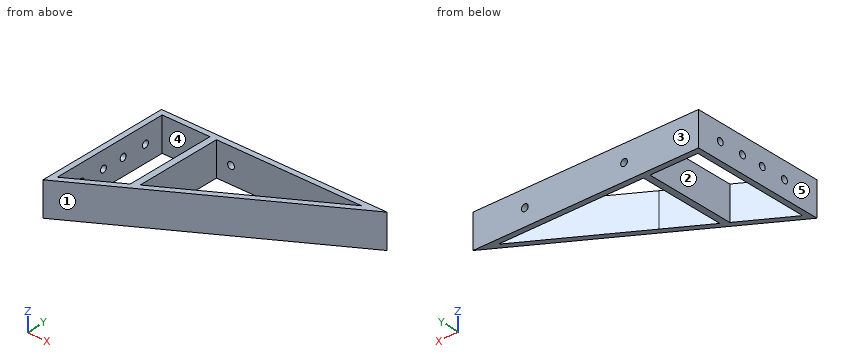
from build123d import *

# Parameters (mm, degrees)
F0_W     = 200
F0_H     = 120
F1_DEPTH = 30
F3_DEPTH = 30
F5_DEPTH = 30
F7_DEPTH = 6
F9_DEPTH = 6


with BuildPart() as f1:
    # F0 (on Top) → F1 (new body)
    with BuildSketch(Plane.XY):
        with Locations((-100, 60)):
            Rectangle(F0_W, F0_H)
    extrude(amount=F1_DEPTH)

    # F2 (on face) → F3 (cut)
    with BuildSketch(Plane.XY.offset(30)):
        Polygon((0, 120), (-200, 0), (0, 0), align=None)
    extrude(amount=-F3_DEPTH, mode=Mode.SUBTRACT)

    # F4 (on face) → F5 (cut)
    with BuildSketch(Plane.XY.offset(30)):
        Polygon((-195, 60.924411), (-195, 8.830952), (-152.64377, 34.24469), (-152.64377, 115), (-195, 115), align=None)
        Polygon((-146.821752, 115), (-146.821752, 37.737901), (-111.472848, 58.947243), (-18.051586, 115), (-115.799665, 115), align=None)
    extrude(amount=-F5_DEPTH, mode=Mode.SUBTRACT)

    # F6 (on face) → F7 (cut)
    with BuildSketch(Plane(origin=(0, 120, 0), x_dir=(-1, 0, 0), z_dir=(0, 1, 0))):
        with BuildLine():
            ThreePointArc((137, 15), (134, 18), (131, 15))
            ThreePointArc((131, 15), (134, 12), (137, 15))
        make_face()
        with BuildLine():
            Line((46, 15), (43, 15))
            ThreePointArc((43, 15), (46, 12), (49, 15))
            Line((49, 15), (46, 15))
        make_face()
        with BuildLine():
            ThreePointArc((49, 15), (46, 18), (43, 15))
            Line((43, 15), (46, 15))
            Line((46, 15), (49, 15))
        make_face()
    extrude(amount=-F7_DEPTH, mode=Mode.SUBTRACT)

    # F8 (on face) → F9 (cut)
    with BuildSketch(Plane(origin=(-200, 0, 0), x_dir=(0, -1, 0), z_dir=(-1, 0, 0))):
        with BuildLine():
            Line((-33, 15), (-30, 15))
            ThreePointArc((-30, 15), (-33, 18), (-36, 15))
            Line((-36, 15), (-33, 15))
        make_face()
        with BuildLine():
            ThreePointArc((-36, 15), (-33, 12), (-30, 15))
            Line((-30, 15), (-33, 15))
            Line((-33, 15), (-36, 15))
        make_face()
        with BuildLine():
            Line((-55.5, 15), (-52.5, 15))
            ThreePointArc((-52.5, 15), (-55.5, 18), (-58.5, 15))
            Line((-58.5, 15), (-55.5, 15))
        make_face()
        with BuildLine():
            ThreePointArc((-58.5, 15), (-55.5, 12), (-52.5, 15))
            Line((-52.5, 15), (-55.5, 15))
            Line((-55.5, 15), (-58.5, 15))
        make_face()
        with BuildLine():
            Line((-75.5, 15), (-72.5, 15))
            ThreePointArc((-72.5, 15), (-75.5, 18), (-78.5, 15))
            Line((-78.5, 15), (-75.5, 15))
        make_face()
        with BuildLine():
            ThreePointArc((-78.5, 15), (-75.5, 12), (-72.5, 15))
            Line((-72.5, 15), (-75.5, 15))
            Line((-75.5, 15), (-78.5, 15))
        make_face()
        with BuildLine():
            ThreePointArc((-95, 15), (-98, 18), (-101, 15))
            Line((-101, 15), (-98, 15))
            Line((-98, 15), (-95, 15))
        make_face()
        with BuildLine():
            Line((-98, 15), (-101, 15))
            ThreePointArc((-101, 15), (-98, 12), (-95, 15))
            Line((-95, 15), (-98, 15))
        make_face()
    extrude(amount=-F9_DEPTH, mode=Mode.SUBTRACT)


solid = f1.part
CAD build for the part. Positions are in the model's coordinates, mm. Face numbers are marked on the shaded views. A direction names the side the tool comes from. Coordinates: 2 decimals unless noted, no trailing zeros. Loops run counter-clockwise (first coordinate to the right, second up) from the corner with the lowest first, then second, coordinate; pieces in that order, holes last. Notation, with made-up numbers: (-20, 5) - (17, 5) arc R12 ccw to (17, 20) - close; hole circle Ø5 at (62.25, 54.5). An arc over 180 degrees is marked (long way). Write item = value, one per line. Start each with the question number.
Q1. Flat gauge pins, fed straight in: pin 1 Ø8 at (y, z) = (65, 12.5) entering from +X; pin 2 Ø5 at (y, z) = (75.5, 15) entering from -X; pin 3 Ø5 at (x, z) = (-46, 15) entering from +Y. Where does each tip first touch, or does it go through?
Q2. Cut at B-B, the plane x = -171. List the corners of the cut face in (y, z), then the cut area to 3 significant figures.
Q3. Cut at C-C, the plane y = 44. List the corners of the cut face in (x, z), then the cut area to 3 significant figures.
Q4. Pull direction Y, two halves, no side cores. Call the marked faces 1, 2 and 3: pulls with the +Y half, pulls with the -Y half, needs draft (parallel to the pull), parting line crosses it, or undercut.
Q5. Cut at A-A, the plane z = 5. List the corners of the cut face in (x, y).
Q6. Which spindle directions (+Z, -Z, +X, -X, +Y, -Y) get a long thin tool onto all of the face, cutting with end or side? Do the marked faces 4 and 5. Say none if no direction does.
Q7. Drill centre lines: L1, parallel to Z at x = -198.8, y = 98; L2, parallel to X at y = 72, z = 21; L3, parallel to X at y = 94, z = 23.5. Where is each one in solid material? Low to high.
Q8. Cut at D-D, the plane x = -134. List the corners of the cut face in (y, z), then the cut area to 3 significant figures.
Computed:
q1.pin_1 = -85
q1.pin_2 = -152.64
q1.pin_3 = 99.73
q2.outline = (17.4, 0) - (23.23, 0) - (23.23, 30) - (17.4, 30) - close; (115, 0) - (120, 0) - (120, 30) - (115, 30) - close
q2.area = 325 mm²
q3.outline = (-200, 0) - (-195, 0) - (-195, 30) - (-200, 30) - close; (-152.64, 0) - (-146.82, 0) - (-146.82, 30) - (-152.64, 30) - close; (-136.38, 0) - (-126.67, 0) - (-126.67, 30) - (-136.38, 30) - close
q3.area = 616 mm²
q4.face_1 = pulls with the -Y half
q4.face_2 = undercut
q4.face_3 = pulls with the +Y half
q5.outline = (-200, 0) - (0, 120) - (-200, 120) - close; hole (-195, 8.83) - (-152.64, 34.24) - (-152.64, 115) - (-195, 115) - close; hole (-146.82, 37.74) - (-18.05, 115) - (-146.82, 115) - close
q6.face_4 = +Z, -Z
q6.face_5 = +Z, -Z, -X, +Y, -Y
q7.L1 = 0 to 12, 18 to 30
q7.L2 = -200 to -195, -152.64 to -146.82, -89.72 to -80
q7.L3 = -200 to -195, -152.64 to -146.82, -53.05 to -43.33
q8.outline = (39.6, 0) - (45.43, 0) - (45.43, 30) - (39.6, 30) - close; (115, 0) - (120, 0) - (120, 12) - (115, 12) - close; (115, 18) - (120, 18) - (120, 30) - (115, 30) - close
q8.area = 295 mm²
